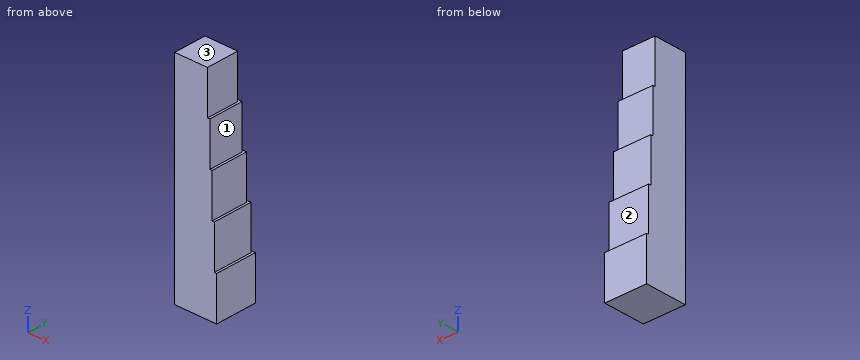
from build123d import *

# Parameters (mm, degrees)
F1_W      = 4.6609
F1_H      = 4.6609
F2_DEPTH  = 4.7625
F3_W      = 4.4069
F3_H      = 4.4069
F4_DEPTH  = 4.7625
F5_W      = 4.1529
F5_H      = 4.1529
F6_DEPTH  = 4.7625
F7_W      = 3.8989
F7_H      = 3.8989
F8_DEPTH  = 4.7625
F9_W      = 3.6449
F9_H      = 3.6449
F10_DEPTH = 4.7625


# Not quite as in the source:
# - a variable given as a bare number and used for a length is read in inches; the dataset says mm whatever the document's units were


with BuildPart() as f2:
    # F1 (on Top) → F2 (new body)
    with BuildSketch(Plane.XY):
        with Locations((2.33045, 2.33045)):
            Rectangle(F1_W, F1_H)
    extrude(amount=F2_DEPTH)

    # F3 (on face) → F4 (join)
    with BuildSketch(Plane.XY.offset(4.7625)):
        with Locations((2.20345, 2.20345)):
            Rectangle(F3_W, F3_H)
    extrude(amount=F4_DEPTH)

    # F5 (on face) → F6 (join)
    with BuildSketch(Plane.XY.offset(9.525)):
        with Locations((2.07645, 2.07645)):
            Rectangle(F5_W, F5_H)
    extrude(amount=F6_DEPTH)

    # F7 (on face) → F8 (join)
    with BuildSketch(Plane.XY.offset(14.2875)):
        with Locations((1.94945, 1.94945)):
            Rectangle(F7_W, F7_H)
    extrude(amount=F8_DEPTH)

    # F9 (on face) → F10 (join)
    with BuildSketch(Plane.XY.offset(19.05)):
        with Locations((1.82245, 1.82245)):
            Rectangle(F9_W, F9_H)
    extrude(amount=F10_DEPTH)


solid = f2.part
For this review, take the finished solid that the model builds, in its own axes (mm). Face numbers are marked on the shaded views. A direction names the side the tool comes from. Coordinates: 2 decimals unless noted, no trailing zeros. Write each loop counter-clockwise with the first axis right and the second up, starting at its lowest first coordinate (ties: lowest second). Pieces come first, ordered by that corner, then holes. Notation, with made-up numbers: (19.25, -26) -> (72.25, -26) arc R15 cw to (72.25, -5) -> close; hole circle Ø3 at (4.5, 85). An arc over 180 degrees is marked (long way). Write each question's results on one line, items separated by ' | '. Start each with the question number.
1) For the marked faces 1, 2 and 3, list the 3-axis set-ups (+Z, -Z, +X, -X, +Y, -Y) from which the entire face can be reached by the end or side of a thin tool; tool diameter is ignored.
2) Consider section C-C (z = 17.5). Write out the cut boundary in (x, y).
3) Wall thickness on L1, parallel to X at y = 3.85, z = 12.75; L2, parallel to Z at x = 0.8, y = 4.2 (3 decimals): over which ranges is each line inside the solid? List them lowest first. Write a range as [from, to].
4) Insertion check: pin 1 (2 mm diameter, centred on y = 3.5, z = 6, fed in from +X); pin 2 (1.8 mm diameter, centred on y = 2.5, z = 21, fed in from +X); pin 3 (1.9 mm diameter, centred on x = 1, z = 16, fed in from +Y); pin 4 (2 mm diameter, centred on y = 4, z = 13, fed in from -X). Each pin has a flat end and moves straight along its axis. Give the tip position at first contact, or say it passes through.
5) Consider section D-D (z = 5.5). Write out the cut boundary in (x, y).
Geometry says:
1) face 1: +Z, +X, +Y, -Y | face 2: +Z, +X, -X, +Y | face 3: +Z, +X, -X, +Y, -Y
2) outline: (0, 0) -> (3.9, 0) -> (3.9, 3.9) -> (0, 3.9) -> close
3) L1: [0, 4.15] | L2: [0, 9.525]
4) pin 1: x = 4.41 | pin 2: x = 3.64 | pin 3: y = 3.9 | pin 4: x = 0
5) outline: (0, 0) -> (4.41, 0) -> (4.41, 4.41) -> (0, 4.41) -> close
